```python
from build123d import *

# Parameters (mm, degrees)
F0_R     = 25
F1_DEPTH = 1000
F2_R     = 35
F3_DEPTH = 25
F5_DEPTH = 1000


with BuildPart() as f1:
    # F0 (on Front) → F1 (new body)
    with BuildSketch(Plane.XZ):
        Circle(F0_R)
    extrude(amount=-F1_DEPTH)

    # F2 (on Top) → F3 (join, symmetric)
    with BuildSketch(Plane.XY):
        with BuildLine():
            Line((25, 0), (-25, 0))
            ThreePointArc((-25, 0), (-45, -37.416574), (-25, -74.833148))
            Line((-25, -74.833148), (25, -74.833148))
            ThreePointArc((25, -74.833148), (45, -37.416574), (25, 0))
        make_face()
        with Locations((0, -37.416574)):
            Circle(F2_R, mode=Mode.SUBTRACT)
    extrude(amount=F3_DEPTH, both=True)

    # F4 (on face) → F5 (join)
    with BuildSketch(Plane.XZ.offset(74.833148)):
        with BuildLine():
            ThreePointArc((0, -25), (17.67767, -17.67767), (25, 0))
            ThreePointArc((25, 0), (17.67767, 17.67767), (0, 25))
            ThreePointArc((0, 25), (-17.67767, 17.67767), (-25, 0))
            ThreePointArc((-25, 0), (-17.67767, -17.677669), (0, -25))
        make_face()
    extrude(amount=F5_DEPTH)


solid = f1.part
```
Can you work these out from the model? Positions are in its coordinate system, mm. A direction names the side the tool comes from. Coordinates: 2 decimals unless noted, no trailing zeros. Write each loop counter-clockwise with the first axis right and the second up, starting at its lowest first coordinate (ties: lowest second). Pieces come first, ordered by that corner, then holes. Notation, with made-up numbers: (37.25, -11.5) - (78.25, -11.5) arc R18 ccw to (78.25, 20.5) - close; hole circle Ø9 at (80, 61.25). An arc over 180 degrees is marked (long way). Return JSON: item names as keys, results as strings.
Q1. If we section it at B-B (y = 554): Please give me the cut outline in (x, z), then the cut area to 3 significant figures.
Computed values:
{"outline": "circle Ø50 at (0, 0)", "area": "1,960 mm2"}
Q2. Please list where these lines run through material, in increasing order: L1, parallel to Y at x = -2, z = -2; L2, parallel to Y at x = 0, z = 12; L3, parallel to Z at x = -0.5, y = 252 (3 decimals). Write a range as from..to.
Computed values:
{"L1": "y = -1074.83..-72.36, -2.47..1000", "L2": "y = -1074.83..-72.42, -2.42..1000", "L3": "z = -24.995..24.995"}
Q3. On a 3-axis mill with a long thin cutter (end or side, diameter ignored), from which of +Z, -Z, +X, -X, +Y, -Y can I reach the whole of each face in a straight line? I mean faces 5 (the cylindrical face through (23.846, 493, 7.509)), 6 (the flat face through (0, -1074.833, 0)). Say none if no direction works.
Computed values:
{"face 5": "+Y", "face 6": "+Z, -Z, +X, -X, -Y"}
Q4. If we section it at A-A (z = -11.5): Please give me the cut outline in (x, y).
Computed values:
{"outline": "(-25, -74.83) - (-22.2, -74.83) - (-22.2, -1074.83) - (22.2, -1074.83) - (22.2, -74.83) - (25, -74.83) arc R45 ccw to (25, 0) - (22.2, 0) - (22.2, 1000) - (-22.2, 1000) - (-22.2, 0) - (-25, 0) arc R45 ccw to start; hole circle Ø70 at (0, -37.42)"}
Q5. Thinking about a two-plate mould opening in Y: for faces 1 (the flat face through (0, 1000, 0)), 2 (the cylindrical face through (44.996, -38.035, 0.35)), 3 (the cylindrical face through (-7.587, -71.584, -0.35)), 4 (the flat face through (-34, -26, 25)), which applies, +Y half, -Y half, draft (parallel to the pull), parting line (faces both ways), or undercut?
Computed values:
{"face 1": "+Y half", "face 2": "parting line", "face 3": "undercut", "face 4": "draft"}
Q6. I'm going to push flat-ended pins straight in: pin 1 Ø5 at (y, z) = (117.5, -8.5) entering from +X; pin 2 Ø5 at (x, z) = (-31.5, -11) entering from -Y; pin 3 Ø5 at (y, z) = (614, -1.5) entering from +X. Where does each tip first touch, or does it pass through?
Computed values:
{"pin 1": "stops at x = 24.27", "pin 2": "stops at y = -71.83", "pin 3": "stops at x = 25"}
